Source: CAD feature listing. Evaluate the final solid. Frame: model axes, mm. A direction names the side the tool comes from. Round coordinates to 2 decimals unless told otherwise and drop trailing zeros. Order: outer loops, then holes, each group sorted by start corner. A loop starts at its lowest first (then second) coordinate and runs counter-clockwise, first axis right, second up. Notation, with made-up numbers: (64, -27.75) -> (101, -27.75) arc R25 cw to (101, -8.75) -> close; hole circle Ø9 at (6, 18.25). An arc over 180 degrees is marked (long way). Answer as CSV lines item,"result".
Autodesk Inventor part; units mm, degrees
ref_plane "YZ Plane" through (0, 0, 0) normal (1, 0, 0) x (0, 1, 0)
ref_plane "XZ Plane" through (0, 0, 0) normal (0, 1, 0) x (-1, 0, 0)
ref_plane "XY Plane" through (0, 0, 0) normal (0, 0, 1) x (1, 0, 0)
sketch "Sketch1" plane through (0, 0, 0) normal (0, 0, 1) x (0, 1, 0)
  line L0 (0, 15) -> (0, -15)
  line L1 (0, -15) -> (6, -15)
  line L2 (6, -15) -> (6, 15)
  line L3 (6, 15) -> (0, 15)
  line L4 (5, 50) -> (0, 50)
  line L5 (0, 50) -> (0, -50)
  line L6 (0, -50) -> (5, -50)
  line L7 (6, -49) -> (6, 49)
  line L8 (-61.2414, 0) -> (17.4485, 0)
  arc A0 (0, 50) -> (0, -50) centre (0, 0) ccw
  arc A1 (0, 44) -> (0, -44) centre (0, 0) ccw
  arc A2 (6, 49) -> (5, 50) centre (5, 49) ccw
  arc A3 (5, -50) -> (6, -49) centre (5, -49) ccw
  dimension "d0" = 30
  dimension "d1" = 6
  dimension "d4" = 100
  dimension "d5" = 6
  dimension "d6" = 1
extrude "Extrusion1" add sketch "Sketch1" along normal blind 100 contours L3 L2 L8 L0 | L8 L2 L1 L0
extrude "Extrusion2" add sketch "Sketch1" along normal blind 6 contours L5 L4 A2 L7 L3 | A1 L8 A0 L5 | L1 L7 A3 L6 L5 | A1 L5 A0 L8
fillet "Fillet1" radius 2 4 edges at (0, 0, 100) (15, 3, 100) (0, 6, 100) (-15, 3, 100)
fillet "Fillet1" radius 1 19 edges at (-15, 0, 53) (-15, 6, 53) (0, 6, 0) (15, 6, 53) (15, 0, 53) (0, 0, 0) (-49.7071, 5.7071, 0) (-50, 2.5, 0) (0, -50, 0) (50, 2.5, 0) (49.7071, 5.7071, 0) (0, -50, 6) (0, -44, 6) (-50, 2.5, 6) (-49.7071, 5.7071, 6) (49.7071, 5.7071, 6) (50, 2.5, 6) (32, 6, 6) (-32, 6, 6)
properties part number "band_stand"
1. Section query B-B on z = 39. Return loops of the section in (x, y), and give its area (3 significant figures).
Results below:
outline,"(-15, 1) arc R1 ccw to (-14, 0) -> (14, 0) arc R1 ccw to (15, 1) -> (15, 5) arc R1 ccw to (14, 6) -> (-14, 6) arc R1 ccw to (-15, 5) -> close"
area,"179 mm2"
2. Section query A-A on x = 0. Return loops of the section in (y, z).
Results below:
outline,"(-50, 1) arc R1 ccw to (-49, 0) -> (-44, 0) -> (-44, 5) arc R1 ccw to (-45, 6) -> (-49, 6) arc R1 ccw to (-50, 5) -> close; (0, 1) arc R1 ccw to (1, 0) -> (5, 0) arc R1 ccw to (6, 1) -> (6, 98) arc R2 ccw to (4, 100) -> (2, 100) arc R2 ccw to (0, 98) -> close"
3. Line query: L1, parallel to Z at x = -25.5, y = -38. Output: solid intervals per line, ascending. Write a range as [from, to].
Results below:
L1,"[0, 6]"
4. Pin query (flat end, axial travel): pin 1 (1.5 mm diameter, centred on x = -12.5, y = -43, fed in from +Z); pin 2 (4.5 mm diameter, centred on y = 3.5, z = 65, fed in from +X); pin 3 (2 mm diameter, centred on y = 4, z = 51, fed in from -X); pin 4 (10 mm diameter, centred on x = 25.5, y = -36, fed in from -Z). Return the tip coordinate at first contact, or that it passes through.
Results below:
pin 1,"z = 6"
pin 2,"x = 15"
pin 3,"x = -15"
pin 4,"z = 0"
5. Reachability of faces 4 (the flat face through (3, 2, 0)), 5 (the flat face through (-1, 0, 38)), 6 (the flat face through (15, 3, 52)) from +Z, -Z, +X, -X, +Y, -Y: full face, straight path, thin tool, end or side. Return the list, or none.
Results below:
face 4,"-Z, +X, -X, +Y, -Y"
face 5,"+Z, -Z"
face 6,"+Z, +X, +Y, -Y"
6. Mould query, pull axis X, two halves, no side actions, for faces 1 (the flat face through (11, -44, 6)), 2 (the cylindrical face through (0.98, -43.99, 2.46)), 3 (the flat face through (-15, 3, 52)). Classes: released by +X, released by -X, zero draft, split by the parting line, or undercut.
Results below:
face 1,"zero draft"
face 2,"undercut"
face 3,"released by -X"
